```python
from build123d import *

# Parameters (mm, degrees)
F0_W     = 1.5524325391
F0_H     = 0.160164271
F0_W_2   = 2.4587620781
F0_H_2   = 0.2921586143
F0_W_3   = 2.2736147407
F0_W_4   = 3.1142332609
F0_W_5   = 2.4696406052
F0_W_6   = 0.6445926557
F1_DEPTH = 2


with BuildPart() as f1:
    # F0 (on Top) → F1 (new body)
    with BuildSketch(Plane.XY):
        Polygon((2.6887415443, 0), (0, 0), (0, -0.4523228854), (0.2299794661, -0.4523228854), (0.2299794661, -0.160164271), (2.6887415443, -0.160164271), align=None)
        Polygon((2.6887415443, 6.0171082268), (2.6887415443, 0), (4.2411740834, 0), (4.2411740834, 4.546245339), (7.3554073443, 4.546245339), (7.3554073443, 6.0171082268), align=None)
        with Locations((3.4649578138, -0.0800821355)):
            Rectangle(F0_W, F0_H)
        with Locations((1.4593605052, -0.3062435782)):
            Rectangle(F0_W_2, F0_H_2)
        Polygon((2.6887415443, -0.4523228854), (0.2299794661, -0.4523228854), (0.2299794661, -2.0985626283), (6.1724845996, -2.0985626283), (6.1724845996, -18.9240246407), (8.3531827515, -18.9240246407), (8.3531827515, -2.0985626283), (14.295687885, -2.0985626283), (14.295687885, -0.4523228854), (12.0220731443, -0.4523228854), (12.0220731443, -1.9231857732), (7.3554073443, -1.9231857732), (2.6887415443, -1.9231857732), align=None)
        Polygon((12.0220731443, 6.0171082268), (7.3554073443, 6.0171082268), (7.3554073443, 4.546245339), (10.4696406052, 4.546245339), (10.4696406052, 0), (12.0220731443, 0), align=None)
        with Locations((11.2458568747, -0.0800821355)):
            Rectangle(F0_W, F0_H)
        with Locations((11.2458568747, -0.3062435782)):
            Rectangle(F0_W, F0_H_2)
        with Locations((13.1588805146, -0.3062435782)):
            Rectangle(F0_W_3, F0_H_2)
        Polygon((8, -0.4523228854), (7.3554073443, -0.4523228854), (7.3554073443, -1.9231857732), (12.0220731443, -1.9231857732), (12.0220731443, -0.4523228854), (10.4696406052, -0.4523228854), align=None)
        Polygon((4.2411740834, -0.4523228854), (2.6887415443, -0.4523228854), (2.6887415443, -1.9231857732), (7.3554073443, -1.9231857732), (7.3554073443, -0.4523228854), align=None)
        with Locations((3.4649578138, -0.3062435782)):
            Rectangle(F0_W, F0_H_2)
        with Locations((5.7982907138, -0.3062435782)):
            Rectangle(F0_W_4, F0_H_2)
        with Locations((9.2348203026, -0.3062435782)):
            Rectangle(F0_W_5, F0_H_2)
        with Locations((7.6777036721, -0.3062435782)):
            Rectangle(F0_W_6, F0_H_2)
    extrude(amount=-F1_DEPTH)


solid = f1.part
```
Check sheet for the modelled part. Datum: model origin and axes. Units: mm. A direction names the side the tool comes from. Round coordinates to 2 decimals unless told otherwise and drop trailing zeros. Loops run counter-clockwise (first coordinate to the right, second up) from the corner with the lowest first, then second, coordinate; pieces in that order, holes last. Notation, with made-up numbers: (81.5, 39) - (117.5, 39) arc R10 cw to (117.5, 46) - close; hole circle Ø7 at (76.5, 35.25). An arc over 180 degrees is marked (long way). Write item = value, one per line. Start each with the question number.
Q1. Section check C-C (x = 7.5). Record the boundary of the cut face in (y, z), plus the area to 3 significant figures.
Q2. Access from +Z, -Z, +X, -X, +Y, -Y to the whole of each face (thin tool, end or side, straight path). Record for faces 5 (the face through (11, -2.099, -1)), 6 (the face through (3, -2.099, -1)), 7 (the face through (4.241, 2, -1)), 8 (the face through (13, -0.16, -1)), 9 (the face through (2.689, 3, -1)).
Q3. Section check A-A (y = 1.5). Record the boundary of the cut face in (x, z), plus the area to 3 significant figures.
Q4. Depth check by flat-ended pin: P1, Ø1, axis at x = 2, z = -0.5, coming from the -Y side; P2, Ø5, axis at x = 8.5, y = -13.5, coming from the +Z side; P3, Ø1, axis at y = 1.5, z = -1, coming from the -X side; P4, Ø0.6, axis at y = -8.5, z = -1, coming from the +X side. Enter the tip coordinate at first touch or a pass-through.
Q5. Section check B-B (z = -1.15). Record the boundary of the cut face in (x, y), plus the area to 3 significant figures.
Q6. Thickness scan on L1, parallel to Y at x = 8.75, z = -0.25; L2, parallel to Y at x = 7, z = -1.85; L3, parallel to X at y = 4.5, z = -1.4. Record the ranges inside material, lowest first.
Q7. Release check for a two-part mould opening along Y. For faces 1 (the face through (8.353, -11, -1)), 2 (the face through (7, -0.16, -1)), 3 (the face through (7, 4.546, -1)), 4 (the face through (1, 0, -1)) record: pulls with the +Y half, pulls with the -Y half, needs draft (parallel to the pull), parting line crosses it, or undercut.
Q8. Section check D-D (x = 11.75). Record the boundary of the cut face in (y, z), plus the area to 3 significant figures.
Derived:
q1.outline = (-18.92, -2) - (-0.16, -2) - (-0.16, 0) - (-18.92, 0) - close; (4.55, -2) - (6.02, -2) - (6.02, 0) - (4.55, 0) - close
q1.area = 40.5 mm^2
q2.face_5 = +Z, -Z, +X, -Y
q2.face_6 = +Z, -Z, -X, -Y
q2.face_7 = +Z, -Z
q2.face_8 = +Z, -Z, +X, +Y
q2.face_9 = +Z, -Z, -X, +Y
q3.outline = (2.69, -2) - (4.24, -2) - (4.24, 0) - (2.69, 0) - close; (10.47, -2) - (12.02, -2) - (12.02, 0) - (10.47, 0) - close
q3.area = 6.21 mm^2
q4.P1 = -2.1
q4.P2 = 0
q4.P3 = 2.69
q4.P4 = 8.35
q5.outline = (0, -0.45) - (0.23, -0.45) - (0.23, -2.1) - (6.17, -2.1) - (6.17, -18.92) - (8.35, -18.92) - (8.35, -2.1) - (14.3, -2.1) - (14.3, -0.16) - (12.02, -0.16) - (12.02, 6.02) - (2.69, 6.02) - (2.69, 0) - (0, 0) - close; hole (4.24, -0.16) - (10.47, -0.16) - (10.47, 4.55) - (4.24, 4.55) - close
q5.area = 92.8 mm^2
q6.L1 = -2.1 to -0.16, 4.55 to 6.02
q6.L2 = -18.92 to -0.16, 4.55 to 6.02
q6.L3 = 2.69 to 4.24, 10.47 to 12.02
q7.face_1 = needs draft
q7.face_2 = undercut
q7.face_3 = undercut
q7.face_4 = pulls with the +Y half
q8.outline = (-2.1, -2) - (6.02, -2) - (6.02, 0) - (-2.1, 0) - close
q8.area = 16.2 mm^2
